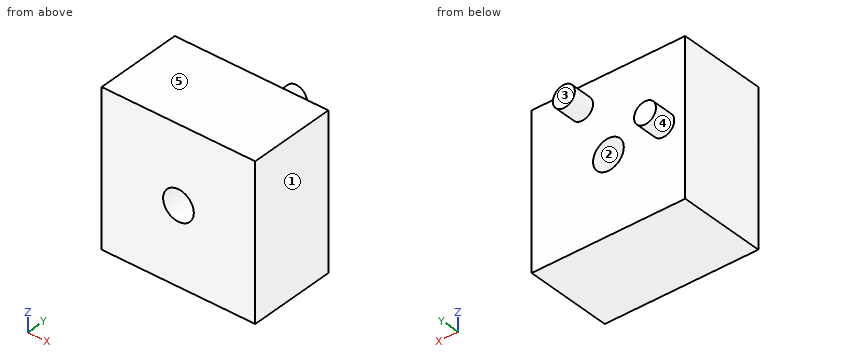
```python
from build123d import *

# Parameters (mm, degrees)
SKETCH1_W           = 44.45
SKETCH1_H           = 44.45
BOSS_EXTRUDE1_DEPTH = 25.4
SKETCH2_R           = 3.175
BOSS_EXTRUDE2_DEPTH = 6.35
SKETCH3_R           = 2.4257
CUT_EXTRUDE1_DEPTH  = 25.4
SKETCH4_R           = 4.445
CUT_EXTRUDE2_DEPTH  = 25.4


with BuildPart() as part:
    # Sketch1 → Boss-Extrude1 (new body)
    with BuildSketch(Plane(origin=(0, 0, 0), x_dir=(1, 0, 0), z_dir=(0, 1, 0))):
        with Locations((22.225, 22.225)):
            Rectangle(SKETCH1_W, SKETCH1_H)
    extrude(amount=BOSS_EXTRUDE1_DEPTH)

    # Sketch2 → Boss-Extrude2 (add)
    with BuildSketch(Plane(origin=(0, 25.4, 0), x_dir=(1, 0, 0), z_dir=(0, 1, 0))):
        with Locations(Location((6.35, 21.59, 0), (0, 0, 270))):
            Circle(SKETCH2_R)
        with Locations(Location((29.845, 6.35, 0), (0, 0, 270))):
            Circle(SKETCH2_R)
    extrude(amount=BOSS_EXTRUDE2_DEPTH)

    # Sketch3 → Cut-Extrude1 (cut)
    with BuildSketch(Plane(origin=(0, 25.4, 0), x_dir=(1, 0, 0), z_dir=(0, 1, 0))):
        with Locations(Location((22.225, 22.225, 0), (0, 0, 270))):
            Circle(SKETCH3_R)
    extrude(amount=-CUT_EXTRUDE1_DEPTH, mode=Mode.SUBTRACT)

    # Sketch4 → Cut-Extrude2 (cut)
    with BuildSketch(Plane.XZ):
        with Locations(Location((22.225, -22.225, 0), (0, 0, 270))):
            Circle(SKETCH4_R)
    extrude(amount=-CUT_EXTRUDE2_DEPTH, mode=Mode.SUBTRACT)


solid = part.part
```
The listing builds one solid part. Answer for the finished solid, in the listing's coordinates (mm). Face numbers are marked on the shaded views. A direction names the side the tool comes from. Give positions to 0.01 mm unless a question says otherwise; leave off trailing zeros. Order: outer loops, then holes, each group sorted by start corner. A loop starts at its lowest first (then second) coordinate and runs counter-clockwise, first axis right, second up. Notation, with made-up numbers: (2, 9) -> (17, 9) arc R32 cw to (17, 39) -> close; hole circle Ø11 at (-2, -2.5). An arc over 180 degrees is marked (long way). Answer as CSV lines item,"result". Start each with the question number.
Q1. Given pin 1 (7 mm diameter, centred on x = 22.225, z = -22.225, fed in from +Y); pin 2 (2 mm diameter, centred on x = 26, z = -13.5, fed in from +Y), each flat-ended and moving along its own axis, determine where each tip first touches the part or whether it passes through.
Q2. A cutting plane is placed at D-D (z = -21.59). Determine the outline of the cut face in (x, y) (3 decimals).
Q3. Determine the mould class of the marked faces 1, 2 and 3 for opening direction X: pulls with the +X half, pulls with the -X half, needs draft (parallel to the pull), parting line crosses it, or undercut.
Q4. A cutting plane is placed at C-C (y = 7). Determine the outline of the cut face in (x, z) (3 decimals), then the cut area to 3 significant figures.
Q5. Find the intervals of material crossed by L1, parallel to Y at x = 15, z = -16.5; L2, parallel to Z at x = 20.5, y = 10.5; L3, parallel to Z at x = 31, y = 29, in increasing order.
Q6. A cutting plane is placed at A-A (z = -6.35). Determine the outline of the cut face in (x, y), then the cut area to 3 significant figures.
Q7. Which of the six approach directions +Z, -Z, +X, -X, +Y, -Y give full straight-line access (tool end or side, diameter ignored) to the marked faces 4 and 5?
Q8. A cutting plane is placed at B-B (x = 6.35). Determine the outline of the cut face in (y, z) (3 decimals), then the cut area to 3 significant figures.
Results found:
1,pin 1,"through"
1,pin 2,"y = 25.4"
2,outline,"(0, 0) -> (17.826, 0) -> (17.826, 25.4) -> (9.525, 25.4) -> (9.525, 31.75) -> (3.175, 31.75) -> (3.175, 25.4) -> (0, 25.4) -> close; (26.624, 0) -> (44.45, 0) -> (44.45, 25.4) -> (26.624, 25.4) -> close"
3,face 1,"pulls with the +X half"
3,face 2,"undercut"
3,face 3,"needs draft"
4,outline,"(0, -44.45) -> (44.45, -44.45) -> (44.45, 0) -> (0, 0) -> close; hole circle Ø8.89 at (22.225, -22.225)"
4,area,"1,910 mm2"
5,L1,"0 to 25.4"
5,L2,"-44.45 to -26.32, -18.13 to 0"
5,L3,"-9.31 to -3.39"
6,outline,"(0, 0) -> (44.45, 0) -> (44.45, 25.4) -> (33.02, 25.4) -> (33.02, 31.75) -> (26.67, 31.75) -> (26.67, 25.4) -> (0, 25.4) -> close"
6,area,"1,170 mm2"
7,face 4,"+Y"
7,face 5,"+Z, +X, -X, +Y, -Y"
8,outline,"(0, -44.45) -> (25.4, -44.45) -> (25.4, -24.765) -> (31.75, -24.765) -> (31.75, -18.415) -> (25.4, -18.415) -> (25.4, 0) -> (0, 0) -> close"
8,area,"1,170 mm2"
